```python
from build123d import *

# Parameters (mm, degrees)
BOSS_EXTRUDE1_DEPTH = 50.8
SKETCH4_R           = 2.54
CUT_EXTRUDE1_DEPTH  = 11.16
SKETCH5_R           = 3.2131
SKETCH5_R_2         = 5.1308
CUT_EXTRUDE2_DEPTH  = 50.8


with BuildPart() as part:
    # Sketch3 → Boss-Extrude1 (new body)
    with BuildSketch(Plane(origin=(0, 0, 0), x_dir=(0, 0, -1), z_dir=(1, 0, 0))):
        Polygon((0, 0), (25.4, 0), (25.4, 25.4), (13.97, 25.4), (13.97, 10.16), (0, 10.16), align=None)
    extrude(amount=-BOSS_EXTRUDE1_DEPTH)

    # Sketch4 → Cut-Extrude1 (cut, through all)
    with BuildSketch(Plane(origin=(0, 10.16, 0), x_dir=(1, 0, 0), z_dir=(0, 1, 0))):
        with Locations((-44.45, 6.35)):
            Circle(SKETCH4_R)
        with Locations((-22.098, 6.35)):
            Circle(SKETCH4_R)
    extrude(amount=-CUT_EXTRUDE1_DEPTH, mode=Mode.SUBTRACT)

    # Sketch5 → Cut-Extrude2 (cut)
    with BuildSketch(Plane.XY.offset(-13.97)):
        with Locations((-38.1, 19.05)):
            Circle(SKETCH5_R)
        with Locations((-12.7, 19.05)):
            Circle(SKETCH5_R_2)
    extrude(amount=-CUT_EXTRUDE2_DEPTH, mode=Mode.SUBTRACT)


solid = part.part
```
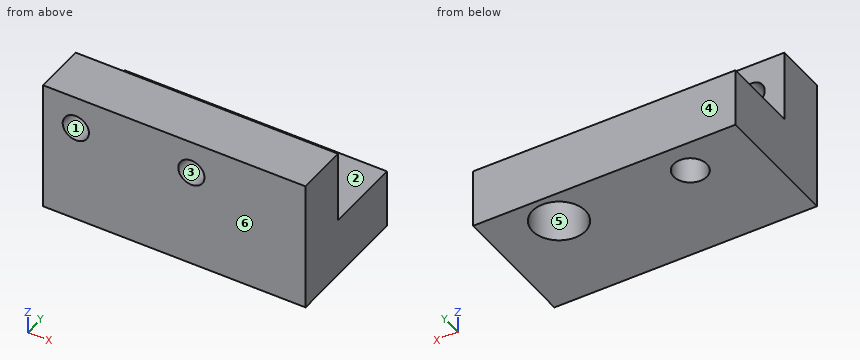
Source: CAD feature listing. Evaluate the final solid. Frame: model axes, mm. Face numbers are marked on the shaded views. A direction names the side the tool comes from. Coordinates: 2 decimals unless noted, no trailing zeros. Order: outer loops, then holes, each group sorted by start corner. A loop starts at its lowest first (then second) coordinate and runs counter-clockwise, first axis right, second up. Notation, with made-up numbers: M 55.5,72 L 97.5,72 A32 cw 97.5,111 Z; hole C 31,38 d4. An arc over 180 degrees is marked long. Write each question's results on one line, items separated by ' | '. Start each with the question number.
1) Section query C-C (z = -6.35). Return the cut outline in (x, y), plus the area to 3 significant figures.
2) Contact query for flat-ended pins moving along their axis: pin 1 Ø11 at (x, z) = (-21, -7.5) entering from +Y; pin 2 Ø12 at (x, y) = (-20.5, 17.5) entering from +Z; pin 3 Ø1.5 at (y, z) = (11, -4) entering from -X. Output: stop coordinate, or through.
3) Draft query along Y for the marked faces 3, 4, 5 and 6. Return one class per face: released by +Y, released by -Y, zero draft, split by the parting line, or undercut.
4) Section query A-A (y = 19.05). Return the cut outline in (x, z).
5) Access query for the marked faces 1 and 2. Directions: +Z, -Z, +X, -X, +Y, -Y. A direction counts if a zero-diameter tool reaches every point of the face in a straight line with its end or side. Return the directions, or none.
6) Line query: line 1 (X direction, y = 2.25, z = -6.35); line 2 (Y direction, x = -38.1, z = -22.5); line 3 (Y direction, x = -12.7, z = -22). Output: solid intervals per line, ascending. Write a range as from..to.
7) Section query B-B (x = -12.7). Return the cut outline in (y, z), plus the area to 3 significant figures.
8) Section query D-D (z = -22.25). Return the cut outline in (x, y).
Answers:
1) outline: M -50.8,0 L -46.99,0 L -46.99,10.16 L -50.8,10.16 Z; M -41.91,0 L -24.64,0 L -24.64,10.16 L -41.91,10.16 Z; M -19.56,0 L 0,0 L 0,10.16 L -19.56,10.16 Z | area: 413 mm^2
2) pin 1: stops at y = 10.16 | pin 2: stops at z = -13.97 | pin 3: passes through
3) face 3: zero draft | face 4: released by +Y | face 5: undercut | face 6: released by -Y
4) outline: M -50.8,-25.4 L -41.31,-25.4 L -41.31,-13.97 L -50.8,-13.97 Z; M -34.89,-25.4 L -17.83,-25.4 L -17.83,-13.97 L -34.89,-13.97 Z; M -7.57,-25.4 L 0,-25.4 L 0,-13.97 L -7.57,-13.97 Z
5) face 1: +Y, -Y | face 2: +Z, +X, -X, +Y
6) line 1: x = -50.8..-46.99, -41.91..-24.64, -19.56..0 | line 2: y = 0..15.84, 22.26..25.4 | line 3: y = 0..13.92, 24.18..25.4
7) outline: M 0,-25.4 L 13.92,-25.4 L 13.92,-13.97 L 10.16,-13.97 L 10.16,0 L 0,0 Z; M 24.18,-25.4 L 25.4,-25.4 L 25.4,-13.97 L 24.18,-13.97 Z | area: 315 mm^2
8) outline: M -50.8,0 L 0,0 L 0,25.4 L -50.8,25.4 Z; hole C -38.1,19.05 d6.43; hole C -12.7,19.05 d10.26
